Build history of the part. All positions in model axes, mm. A direction names the side the tool comes from. Give positions to 0.01 mm unless a question says otherwise; leave off trailing zeros. Order: outer loops, then holes, each group sorted by start corner. A loop starts at its lowest first (then second) coordinate and runs counter-clockwise, first axis right, second up. Notation, with made-up numbers: M 29,55.25 L 62,55.25 A18 ccw 62,72.25 Z; hole C 58.25,-27.5 d2. An arc over 180 degrees is marked long. Use CSV: the item, a comma, the result in double quotes. Start each with the question number.
Item 1: Band-saw the part on A-A on z = 0. Write the cut outline in (x, y).
Item 2: Two-plate mould, pull along Z, no slides. Class faces 4 (the cylindrical face through (7.684, -2.014, 1.009)), 5 (the flat face through (-6, 5, 12)), 6 (the cylindrical face through (-24.397, 2.465, 12.69)): pulls with the +Z half, pulls with the -Z half, needs draft (parallel to the pull), parting line crosses it, or undercut.
Item 3: Which spindle directions (+Z, -Z, +X, -X, +Y, -Y) get a long thin tool onto all of the face, cutting with end or side? Do faces 1 (the cylindrical face through (-17.007, 2.465, 11.575)), 2 (the flat face through (-12, 0, 0)), 3 (the flat face through (3, 6, 1)). Say none if no direction does.
Item 4: Band-saw the part on D-D on y = 23. Write the cut outline in (x, z).
Item 5: Band-saw the part on C-C on x = 18.5. Write the cut outline in (y, z).
Item 6: Pin check, flat tips, straight feed: P1, Ø10, axis at x = 3, y = 17, coming from the -Z side; P2, Ø3, axis at x = 0, z = 22.5, coming from the -Y side; P3, Ø3, axis at y = 21.5, z = -3, coming from the +X side; P4, Ø5, axis at x = -7.5, y = 15.5, coming from the +Z side. Stop position of each tip, or through.
Item 7: Wall check: line 1 along X through (y, z) = (3, 0); line 2 along X through (y, z) = (-2.3, 0); line 3 along X through (y, z) = (1.6, 11.25). Give the ranges that are in metal, low to high.
Item 8: Band-saw the part on B-B on z = 11.5. Write the cut outline in (x, y), plus the area to 3 significant figures.
from build123d import *

# Parameters (mm, degrees)
SKETCH_1_R          = 27.5
EXTRUDE_1_DEPTH     = 5
SKETCH_2_R          = 10
EXTRUDE_2_DEPTH     = 3
SKETCH_3_R          = 13
EXTRUDE_3_DEPTH     = 23
SKETCH_4_R          = 6
CUT_EXTRUDE_1_DEPTH = 22
SKETCH_5_R          = 7.75
CUT_EXTRUDE_2_DEPTH = 2
SKETCH_6_R          = 3
CUT_EXTRUDE_3_DEPTH = 49.512884886
SKETCH_7_R          = 2.5
CUT_EXTRUDE_4_DEPTH = 48.921811318


with BuildPart() as part:
    # 草图1 → 凸台-拉伸1 (new body)
    with BuildSketch(Plane(origin=(0, 0, 0), x_dir=(1, 0, 0), z_dir=(0, 1, 0))):
        with Locations(Location((0, 0, 0), (0, 0, 270))):
            Circle(SKETCH_1_R)
    extrude(amount=EXTRUDE_1_DEPTH)

    # 草图2 → 凸台-拉伸2 (add)
    with BuildSketch(Plane.XZ):
        with Locations(Location((0, 0, 0), (0, 0, 270))):
            Circle(SKETCH_2_R)
    extrude(amount=EXTRUDE_2_DEPTH)

    # 草图3 → 凸台-拉伸3 (add)
    with BuildSketch(Plane(origin=(0, 5, 0), x_dir=(1, 0, 0), z_dir=(0, 1, 0))):
        with Locations(Location((0, 0, 0), (0, 0, 270))):
            Circle(SKETCH_3_R)
    extrude(amount=EXTRUDE_3_DEPTH)

    # 草图4 → 切除-拉伸1 (cut)
    with BuildSketch(Plane(origin=(0, 28, 0), x_dir=(1, 0, 0), z_dir=(0, 1, 0))):
        with Locations(Location((0, 0, 0), (0, 0, 270))):
            Circle(SKETCH_4_R)
    extrude(amount=-CUT_EXTRUDE_1_DEPTH, mode=Mode.SUBTRACT)

    # 草图5 → 切除-拉伸2 (cut)
    with BuildSketch(Plane.XZ.offset(3)):
        with Locations(Location((0, 0, 0), (0, 0, 270))):
            Circle(SKETCH_5_R)
    extrude(amount=-CUT_EXTRUDE_2_DEPTH, mode=Mode.SUBTRACT)

    # 草图6 → 切除-拉伸3 (cut, through all)
    with BuildSketch(Plane.XZ.offset(1)):
        with Locations(Location((0, 0, 0), (0, 0, 270))):
            Circle(SKETCH_6_R)
    extrude(amount=-CUT_EXTRUDE_3_DEPTH, mode=Mode.SUBTRACT)

    # 草图7 → 切除-拉伸4 (cut, through all)
    with BuildSketch(Plane.XZ):
        with Locations(Location((0, 22.5, 0), (0, 0, 270))):
            Circle(SKETCH_7_R)
        with Locations(Location((19.485571585, 11.25, 0), (0, 0, 270))):
            Circle(SKETCH_7_R)
        with Locations(Location((19.485571585, -11.25, 0), (0, 0, 270))):
            Circle(SKETCH_7_R)
        with Locations(Location((0, -22.5, 0), (0, 0, 270))):
            Circle(SKETCH_7_R)
        with Locations(Location((-19.485571585, -11.25, 0), (0, 0, 270))):
            Circle(SKETCH_7_R)
        with Locations(Location((-19.485571585, 11.25, 0), (0, 0, 270))):
            Circle(SKETCH_7_R)
    extrude(amount=-CUT_EXTRUDE_4_DEPTH, mode=Mode.SUBTRACT)


solid = part.part
Model answer:
1,outline,"M -27.5,0 L -10,0 L -10,-3 L -7.75,-3 L -7.75,-1 L -3,-1 L -3,6 L -6,6 L -6,28 L -13,28 L -13,5 L -27.5,5 Z; M 3,-1 L 7.75,-1 L 7.75,-3 L 10,-3 L 10,0 L 27.5,0 L 27.5,5 L 13,5 L 13,28 L 6,28 L 6,6 L 3,6 Z"
2,face 4,"undercut"
2,face 5,"needs draft"
2,face 6,"parting line crosses it"
3,face 1,"+Y, -Y"
3,face 2,"-Y"
3,face 3,"+Y"
4,outline,"C 0,0 d26; hole C 0,0 d12"
5,outline,"M 0,-20.35 L 5,-20.35 L 5,-13.55 L 0,-13.55 Z; M 0,-8.95 L 5,-8.95 L 5,8.95 L 0,8.95 Z; M 0,13.55 L 5,13.55 L 5,20.35 L 0,20.35 Z"
6,P1,"stops at z = -13"
6,P2,"passes through"
6,P3,"stops at x = 12.91"
6,P4,"stops at z = 12"
7,line 1,"x = -27.5 to -3, 3 to 27.5"
7,line 2,"x = -10 to -7.75, 7.75 to 10"
7,line 3,"x = -25.09 to -21.99, -16.99 to 16.99, 21.99 to 25.09"
8,outline,"M -24.98,0 L -21.97,0 L -21.97,5 L -24.98,5 Z; M -17,0 L 17,0 L 17,5 L 6.06,5 L 6.06,28 L -6.06,28 L -6.06,5 L -17,5 Z; M 21.97,0 L 24.98,0 L 24.98,5 L 21.97,5 Z"
8,area,"479 mm^2"
